Design review of the part built by this model. Coordinates are the model's own, in mm. A direction names the side the tool comes from. Round coordinates to 2 decimals unless told otherwise and drop trailing zeros. Write each loop counter-clockwise with the first axis right and the second up, starting at its lowest first coordinate (ties: lowest second). Pieces come first, ordered by that corner, then holes. Notation, with made-up numbers: (47.5, -1.75) - (64.5, -1.75) arc R20 ccw to (64.5, 13.25) - close; hole circle Ø9 at (54, 32.25). An arc over 180 degrees is marked (long way). Use one line per item in the form item = value.
Autodesk Inventor part; units mm, degrees
ref_plane "YZ Plane" through (0, 0, 0) normal (1, 0, 0) x (0, 1, 0)
ref_plane "XZ Plane" through (0, 0, 0) normal (0, 1, 0) x (-1, 0, 0)
ref_plane "XY Plane" through (0, 0, 0) normal (0, 0, 1) x (1, 0, 0)
sketch "Sketch1" plane through (0, 0, 0) normal (0, 0, 1) x (1, 0, 0)
  circle A0 centre (0, 0) radius 32.5
  dimension "d0" = 65
extrude "Extrusion1" add sketch "Sketch1" along normal blind 58
sketch "Sketch2" plane through (0, 0, 58) normal (0, 0, 1) x (1, 0, 0)
  circle A0 centre (0, 0) radius 24.2
  dimension "d3" = 48.4
extrude "Extrusion2" cut sketch "Sketch2" against normal blind 30
sketch "Sketch3" plane through (0, 0, 0) normal (0, 0, -1) x (-1, 0, 0)
  circle A0 centre (0, 0) radius 12.15
  dimension "d6" = 24.3
extrude "Extrusion3" cut sketch "Sketch3" against normal through all
sketch "Sketch4" plane through (0, 0, 0) normal (0, 0, -1) x (-1, 0, 0)
  circle A0 centre (0, 0) radius 16 construction
  point P0 (-16, 0)
  point P1 (16, 0)
  point P2 (0, -16)
  point P3 (0, 16)
  dimension "d9" = 32
hole "Hole1" at (16, 0, 0) at (-16, 0, 0) at (0, -16, 0) at (0, 16, 0) direction (0, 0, 1) diameter 3 depth 10 tip angle 80
chamfer "Chamfer1" distance 1 angle 45 4 edges at (-32.5, 0, 58) (12.15, 0, 0) (-24.2, 0, 58) (12.15, 0, 28)
chamfer "Chamfer2" distance 0.4 angle 45 1 edges at (-24.2, 0, 28)
chamfer "Chamfer3" distance 12 angle 70 1 edges at (-32.5, 0, 0) measured on face at (9.1116, -18.0337, 0)
chamfer "Chamfer4" distance 0.4 angle 45 4 edges at (0, -17.5, 0) (-16, -1.5, 0) (16, -1.5, 0) (0, 14.5, 0)
properties part number "FujiiEchelleColilmatorAttachement" material "ABS Plastic"
Q1. Machinability: for faces 1 (the cylindrical face through (2.63, -11.86, 13.82)), 2 (the cylindrical face through (17.464, -0.325, 5.267)), 3 (the cylindrical face through (22.355, -9.269, 42.9)), which of the approach directions +Z, -Z, +X, -X, +Y, -Y give a long, thin tool a straight path to every point of the face, cutting with its end or side? Answer none if there is none.
Calculated:
face_1 = +Z, -Z
face_2 = -Z
face_3 = +Z
Q2. We need section A-A on z = 52. Write out the cut boundary in (x, y), then the cut area to 3 significant figures.
Calculated:
outline = circle Ø65 at (0, 0); hole circle Ø48.4 at (0, 0)
area = 1,480 mm2
Q3. To check wall thickness, follow line 1 along X through (y, z) = (-16, 3); line 2 along Y through (x, z) = (0, 5); line 3 along Y through (x, z) = (0, 6.25). State the ranges of each line that lie inside material, in increasing order. Write a range as from..to.
Calculated:
line_1 = -14.5..-1.5, 1.5..14.5
line_2 = -22.32..-17.5, -14.5..-12.15, 12.15..14.5, 17.5..22.32
line_3 = -22.77..-17.5, -14.5..-12.15, 12.15..14.5, 17.5..22.77
Q4. For P1, Ø14.5, axis at x = 9.5, y = -8.5, coming from the +Z side; P2, Ø2.5, axis at x = 0, y = -16, coming from the -Z side; P3, Ø1, axis at y = 17, z = 7, coming from the +X side, all flat-tipped, find the tip position at first contact; note any pin that passes through.
Calculated:
P1 = 28
P2 = 10.3
P3 = 16.15
Q5. Draft analysis for pull direction Y (two halves, no side actions). For faces 4 (the conical face through (-18.98, -14.553, 9.389)), 5 (the cylindrical face through (-17.01, -1.11, 5.27)), 6 (the flat face through (-0.3, -13.4, 0)), state which applies: released by +Y, released by -Y, zero draft, split by the parting line, or undercut.
Calculated:
face_4 = split by the parting line
face_5 = undercut
face_6 = zero draft
